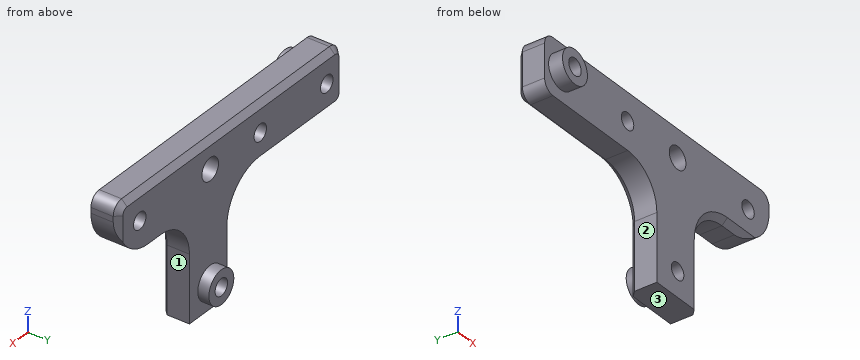
```python
from build123d import *

# Parameters (mm, degrees)
SKETCH1_W           = 54
SKETCH1_H           = 10
BOSS_EXTRUDE1_DEPTH = 5
SKETCH3_R           = 1.5
SKETCH3_R_2         = 2
CUT_EXTRUDE1_DEPTH  = 7
FILLET1_R           = 2
SKETCH4_R           = 3
SKETCH4_R_2         = 1.5
BOSS_EXTRUDE2_DEPTH = 2.5
SKETCH5_W           = 10
SKETCH5_H           = 5
BOSS_EXTRUDE3_DEPTH = 19
SKETCH6_R           = 1.5
CUT_EXTRUDE2_DEPTH  = 10
BOSS_EXTRUDE4_START = 2
SKETCH7_R           = 3
SKETCH7_R_2         = 1.5
BOSS_EXTRUDE4_DEPTH = 2
FILLET2_R           = 7
CHAMFER1_SIZE       = 1
FILLET3_R           = 7


with BuildPart() as part:
    # Sketch1 → Boss-Extrude1 (new body)
    with BuildSketch(Plane(origin=(0, 0, 0), x_dir=(1, 0, 0), z_dir=(0, 1, 0))):
        Rectangle(SKETCH1_W, SKETCH1_H)
    extrude(amount=BOSS_EXTRUDE1_DEPTH)

    # Sketch3 → Cut-Extrude1 (cut)
    with BuildSketch(Plane(origin=(0, 5, 0), x_dir=(1, 0, 0), z_dir=(0, 1, 0))):
        with Locations(Location((-23.05, 0, 0), (0, 0, 270))):
            Circle(SKETCH3_R)
        with Locations(Location((5, 0, 0), (0, 0, 270))):
            Circle(SKETCH3_R_2)
        with Locations(Location((-7.05, 0, 0), (0, 0, 270))):
            Circle(SKETCH3_R)
        with Locations(Location((21.95, 0, 0), (0, 0, 270))):
            Circle(SKETCH3_R)
    extrude(amount=-CUT_EXTRUDE1_DEPTH, mode=Mode.SUBTRACT)

    # Fillet1
    fillet1_edges = [part.edges().sort_by_distance(p)[0] for p in [
        (27, 2.5, 5),
        (-27, 2.5, 5),
        (-27, 2.5, -5),
    ]]
    fillet(fillet1_edges, radius=FILLET1_R)

    # Sketch4 → Boss-Extrude2 (add)
    with BuildSketch(Plane.XZ):
        with Locations(Location((-23.05, 0, 0), (0, 0, 270))):
            Circle(SKETCH4_R)
        with Locations(Location((-23.05, 0, 0), (0, 0, 90))):
            Circle(SKETCH4_R_2, mode=Mode.SUBTRACT)
    extrude(amount=BOSS_EXTRUDE2_DEPTH)

    # Sketch5 → Boss-Extrude3 (add)
    with BuildSketch(Plane(origin=(0, 0, -5), x_dir=(-1, 0, 0), z_dir=(0, 0, -1))):
        with Locations((-5, 2.5)):
            Rectangle(SKETCH5_W, SKETCH5_H)
    extrude(amount=BOSS_EXTRUDE3_DEPTH)

    # Sketch6 → Cut-Extrude2 (cut)
    with BuildSketch(Plane(origin=(0, 5, 0), x_dir=(1, 0, 0), z_dir=(0, 1, 0))):
        with Locations(Location((5, 19.5, 0), (0, 0, 270))):
            Circle(SKETCH6_R)
    extrude(amount=-CUT_EXTRUDE2_DEPTH, mode=Mode.SUBTRACT)

    # Sketch7 → Boss-Extrude4 (add)
    with BuildSketch(Plane(origin=(0, 5, 0), x_dir=(1, 0, 0), z_dir=(0, 1, 0)).offset(BOSS_EXTRUDE4_START)):
        with Locations(Location((5, 19.5, 0), (0, 0, 270))):
            Circle(SKETCH7_R)
        with Locations(Location((5, 19.5, 0), (0, 0, 270))):
            Circle(SKETCH7_R_2, mode=Mode.SUBTRACT)
    extrude(amount=-BOSS_EXTRUDE4_DEPTH)

    # Fillet2
    fillet2_edges = [part.edges().sort_by_distance(p)[0] for p in [
        (10, 2.5, -5),
        (0, 2.5, -5),
    ]]
    fillet(fillet2_edges, radius=FILLET2_R)

    # Chamfer1
    chamfer1_edges = [part.edges().sort_by_distance(p)[0] for p in [
        (10, 0, -18),
        (12.050252532, 0, -7.050252532),
        (22, 0, -5),
        (0, 5, -18),
        (-2.050252532, 5, -7.050252532),
        (-16, 5, -5),
        (-26.414213562, 5, -4.414213562),
        (-27, 5, 0),
        (-26.414213562, 5, 4.414213562),
        (0, 5, 5),
        (26.414213562, 5, 4.414213562),
        (27, 5, -1),
    ]]
    chamfer(chamfer1_edges, length=CHAMFER1_SIZE)

    # Fillet3
    fillet3_edges = [part.edges().sort_by_distance(p)[0] for p in [
        (27, 2.5, -5),
    ]]
    fillet(fillet3_edges, radius=FILLET3_R)


solid = part.part
```
Part model, mm, in its own coordinate system. Face numbers are marked on the shaded views. A direction names the side the tool comes from. Round coordinates to 2 decimals unless told otherwise and drop trailing zeros. Write each loop counter-clockwise with the first axis right and the second up, starting at its lowest first coordinate (ties: lowest second). Pieces come first, ordered by that corner, then holes. Notation, with made-up numbers: (46.25, -16.5) -> (97.25, -16.5) arc R36 ccw to (97.25, 20.5) -> close; hole circle Ø11 at (-23, 4.25). An arc over 180 degrees is marked (long way). Return JSON: item names as keys, results as strings. Group by question number.
Q1. Saw through at D-D on x = -22.5. Write the cut outline in (y, z), plus the area to 3 significant figures.
Q2. Pin check, flat tips, straight feed: pin 1 (2.5 mm diameter, centred on x = -23.05, z = 0, fed in from -Y); pin 2 (5 mm diameter, centred on x = -17.5, y = -1, fed in from -Z); pin 3 (1 mm diameter, centred on x = -4.5, y = 1, fed in from -Z); pin 4 (4.5 mm diameter, centred on y = 2.5, z = -19, fed in from +X). Stop position of each tip, or through.
Q3. Saw through at A-A on x = 5. Write the cut outline in (y, z), plus the area to 4 significant figures.
Q4. Saw through at C-C on z = 0.75. Write the cut outline in (x, y).
Q5. Probe L1, parallel to X at y = 3.5, z = -19.5; L2, parallel to Z at x = 4, y = 4.75; L3, parallel to Z at x = -23.05, y = 3.5. List the from-to ranges inside material, lowest first. Write a range as [from, to].
Q6. Saw through at B-B on z = -19.5. Write the cut outline in (x, y).
Q7. Which spindle directions (+Z, -Z, +X, -X, +Y, -Y) get a long thin tool onto all of the face, cutting with end or side? Do the marked faces 1, 2 and 3. Say none if no direction does.
Answer:
{
 "1": {"outline": "(-2.5, -2.95) -> (0, -2.95) -> (0, -5) -> (4, -5) -> (5, -4) -> (5, -1.4) -> (-2.5, -1.4) -> close; (-2.5, 1.4) -> (5, 1.4) -> (5, 4) -> (4, 5) -> (0, 5) -> (0, 2.95) -> (-2.5, 2.95) -> close", "area": "42.8 mm2"},
 "2": {"pin 1": "through", "pin 2": "z = -5", "pin 3": "z = -5.68", "pin 4": "x = 10"},
 "3": {"outline": "(0, -24) -> (5, -24) -> (5, -22.5) -> (7, -22.5) -> (7, -21) -> (0, -21) -> close; (0, -18) -> (7, -18) -> (7, -16.5) -> (5, -16.5) -> (5, -2) -> (0, -2) -> close; (0, 2) -> (5, 2) -> (5, 4) -> (4, 5) -> (0, 5) -> close", "area": "115.5 mm2"},
 "4": {"outline": "(-27, 0) -> (-25.95, 0) -> (-25.95, -2.5) -> (-24.35, -2.5) -> (-24.35, 5) -> (-26, 5) -> (-27, 4) -> close; (-21.75, -2.5) -> (-20.15, -2.5) -> (-20.15, 0) -> (-8.35, 0) -> (-8.35, 5) -> (-21.75, 5) -> close; (-5.75, 0) -> (3.15, 0) -> (3.15, 5) -> (-5.75, 5) -> close; (6.85, 0) -> (20.65, 0) -> (20.65, 5) -> (6.85, 5) -> close; (23.25, 0) -> (26.89, 0) -> (26.89, 4.11) -> (26, 5) -> (23.25, 5) -> close"},
 "5": {"L1": "[0, 3.5], [6.5, 10]", "L2": "[-24, -20.62], [-18.38, -1.73], [1.73, 4.25]", "L3": "[-5, -1.5], [1.5, 5]"},
 "6": {"outline": "(0, 0) -> (3.5, 0) -> (3.5, 7) -> (2, 7) -> (2, 5) -> (1, 5) -> (0, 4) -> close; (6.5, 0) -> (9, 0) -> (10, 1) -> (10, 5) -> (8, 5) -> (8, 7) -> (6.5, 7) -> close"},
 "7": {"face 1": "-Z, +X, +Y, -Y", "face 2": "-Z, -X, +Y, -Y", "face 3": "-Z, +X, -X, +Y, -Y"}
}
